Source: CAD feature listing. Evaluate the final solid. Frame: model axes, mm. Face numbers are marked on the shaded views. Give positions to 0.01 mm unless a question says otherwise; leave off trailing zeros. Loops run counter-clockwise (first coordinate to the right, second up) from the corner with the lowest first, then second, coordinate; pieces in that order, holes last. Notation, with made-up numbers: (17, 89.5) -> (63, 89.5) arc R12 cw to (63, 107.5) -> close; hole circle Ø7 at (44, 68.5). An arc over 180 degrees is marked (long way). Answer as a JSON object with one key per item and string values. Group by question number.
from build123d import *

# Parameters (mm, degrees)
F0_R     = 7.5
F0_R_2   = 2.5
F1_DEPTH = 21
F2_R     = 6
F2_R_2   = 1.651
F3_DEPTH = 15
F5_D     = 2.7
F5_DEPTH = 7.501
F6_D     = 2.7
F7_SIZE  = 0.5


with BuildPart() as f1:
    # F0 (on Top) → F1 (new body)
    with BuildSketch(Plane.XY):
        Circle(F0_R)
        Circle(F0_R_2, mode=Mode.SUBTRACT)
    extrude(amount=F1_DEPTH)

    # F2 (on face) → F3 (join)
    with BuildSketch(Plane.XY.offset(21)):
        Circle(F2_R)
        Circle(F2_R_2, mode=Mode.SUBTRACT)
    extrude(amount=F3_DEPTH)

    # F5 (through all, one way)
    with BuildSketch(Plane.XZ):
        with Locations((0, 5), (0, 31)):
            Circle(F5_D / 2)
    extrude(amount=-F5_DEPTH, mode=Mode.SUBTRACT)

    # F6 (through all)
    with Locations(Plane(origin=(0, 0, 0), x_dir=(1, 0, 0), z_dir=(0, 1, 0))):
        with Locations((0, -5), (0, -31)):
            Hole(F6_D / 2)

    # F7
    f7_edges = [f1.edges().sort_by_distance(p)[0] for p in [
        (-7.5, 0, 0),
        (-7.5, 0, 21),
        (-6, 0, 36),
        (-2.5, 0, 0),
        (-6, 0, 21),
        (-2.5, 0, 21),
        (-1.651, 0, 36),
    ]]
    chamfer(f7_edges, length=F7_SIZE)


solid = f1.part
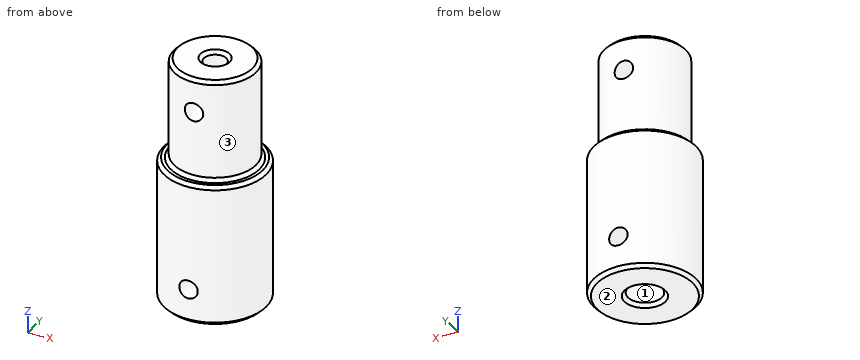
(1) Material intervals for line 1 (Z direction, x = 0, y = -3.8); line 2 (Y direction, x = 0, z = 23); line 3 (X direction, y = -4.3, z = 5), sorted ascending. Write a range as from..to.
(2) Section query C-C on x = 0. State how many separate pieces and enclosed holes the cut face has, plus the area to 3 significant figures.
(3) Mould query, pull axis Y, two halves, no side actions, for the marked faces 1, 2 and 3. Classes: pulls with the +Y half, pulls with the -Y half, needs draft (parallel to the pull), parting line crosses it, or undercut.
(4) Section query B-B on z = 5. Return the cut outline in (x, y).
(5) First-contact query: pin 1 (3.5 mm diameter, centred on x = 0, z = 5, fed in from -Y); pin 2 (1.5 mm diameter, centred on y = 3.5, z = 24, fed in from -X); pin 3 (3 mm diameter, centred on x = 0, y = 0, fed in from -Z); pin 4 (1 mm diameter, centred on y = 5, z = 23.5, fed in from -X). Flat tips, straight axial feed; report the tip coordinate or a pass-through.
(6) Section query D-D on z = 18. Return the cut outline in (x, y), plus the area to 3 significant figures.
Result:
{
 "1": {"line 1": "0..3.65, 6.35..29.65, 32.35..36", "line 2": "-6..-1.65, 1.65..6", "line 3": "-6.14..-1.35, 1.35..6.14"},
 "2": {"separate pieces": "6", "enclosed holes": "0", "area": "289 mm²"},
 "3": {"face 1": "undercut", "face 2": "needs draft", "face 3": "parting line crosses it"},
 "4": {"outline": "(-1.35, -7.38) -> (-1.35, -2.1) arc R2.5 cw to (-1.35, 2.1) -> (-1.35, 7.38) arc R7.5 ccw to start; (1.35, -7.38) arc R7.5 ccw to (1.35, 7.38) -> (1.35, 2.1) arc R2.5 cw to (1.35, -2.1) -> close"},
 "5": {"pin 1": "y = -7.5", "pin 2": "x = -5.33", "pin 3": "through", "pin 4": "x = -3.97"},
 "6": {"outline": "circle Ø15 at (0, 0); hole circle Ø5 at (0, 0)", "area": "157 mm²"}
}
